Verification items for the finished model (mm, model axes). Face numbers are marked on the shaded views. A direction names the side the tool comes from. Coordinates: 2 decimals unless noted, no trailing zeros. Write each loop counter-clockwise with the first axis right and the second up, starting at its lowest first coordinate (ties: lowest second). Pieces come first, ordered by that corner, then holes. Notation, with made-up numbers: (-15.5, 77.5) -> (28.5, 77.5) arc R24 ccw to (28.5, 89.5) -> close; hole circle Ø3 at (8.5, -25). An arc over 180 degrees is marked (long way). Answer in a Markdown table with one row per item.
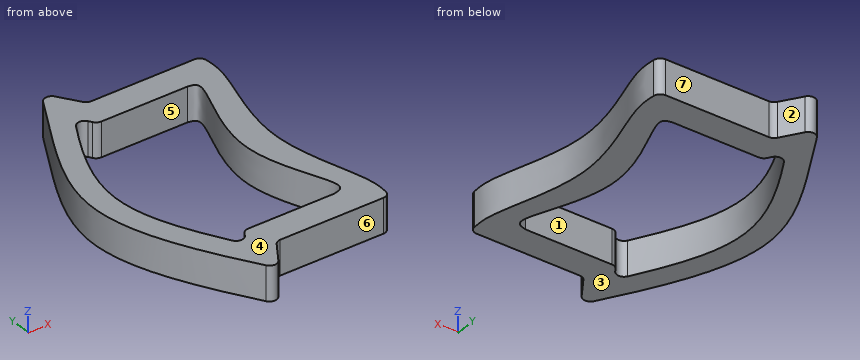
```python
from build123d import *

# Parameters (mm, degrees)
F1_DEPTH = 19.05
F3_DEPTH = 19.05
F4_R     = 4


with BuildPart() as f1:
    # F0 (on Top) → F1 (new body)
    with BuildSketch(Plane.XY):
        with BuildLine():
            add(Edge.make_bspline(
                [(0, -88.9), (-18.7615667395, -58.872751179), (-55.497587887, 2.319356984), (-18.3044684192, 54.234037211), (0, 88.9)],
                knots=[0, 0, 0, 0, 0.5, 1, 1, 1, 1], degree=3))
            Line((0, -88.9), (12.096735135, -70.5242279326))
            Line((12.096735135, -70.5242279326), (75.096735135, -70.5242279326))
            add(Edge.make_bspline(
                [(75.096735135, 70.5242279326), (75.6453777141, 65.842621729), (77.7669512859, 52.4624280909), (54.0778767649, 0.0958361046), (77.7020868907, -53.1321501243), (75.6250650534, -66.0721629988), (75.096735135, -70.5242279326)],
                knots=[0, 0, 0, 0, 0.1764310118, 0.500837432, 0.8270944973, 1, 1, 1, 1], degree=3))
            Line((75.096735135, 70.5242279326), (12.096735135, 70.5242279326))
            Line((12.096735135, 70.5242279326), (0, 88.9))
        make_face()
    extrude(amount=F1_DEPTH)

    # F2 (on face) → F3 (cut)
    with BuildSketch(Plane.XY.offset(19.05)):
        with BuildLine():
            add(Edge.make_bspline(
                [(0, -63.9), (-15.0066513258, -38.561437128), (-33.4891316908, -0.0640391576), (-15.0195212491, 38.6895154432), (0, 63.9)],
                knots=[0, 0, 0, 0, 0.5, 1, 1, 1, 1], degree=3))
            Line((0, -63.9), (6.0483675675, -54.7121139663))
            Line((6.0483675675, -54.7121139663), (56.0483675675, -54.7121139663))
            add(Edge.make_bspline(
                [(55.7842407716, 54.5435819516), (57.8413429651, 54.264139175), (66.4918207205, 53.0890329839), (32.3838227626, -0.5635362626), (68.3251031662, -51.8911242436), (58.5903282755, -54.1280136592), (56.0483675675, -54.7121139663)],
                knots=[0, 0, 0, 0, 0.1173857138, 0.4936276425, 0.8677752027, 1, 1, 1, 1], degree=3))
            Line((55.7842407716, 54.5435819516), (5.7842407716, 54.5435819516))
            Line((5.7842407716, 54.5435819516), (0, 63.9))
        make_face()
    extrude(amount=-F3_DEPTH, mode=Mode.SUBTRACT)

    # F4
    f4_edges = [f1.edges().sort_by_distance(p)[0] for p in [
        (0, -88.9, 9.525),
        (75.096735, -70.524228, 9.525),
        (5.784241, 54.543582, 9.525),
        (75.096735, 70.524228, 9.525),
        (0, 88.9, 9.525),
        (12.096735, 70.524228, 9.525),
        (12.096735, -70.524228, 9.525),
        (0, 63.9, 9.525),
        (0, -63.9, 9.525),
        (6.048368, -54.712114, 9.525),
    ]]
    fillet(f4_edges, radius=F4_R)


solid = f1.part
```
1. Go/stop test with flat-tipped pins: pin 1 (1.5 mm diameter, centred on y = 28.5, z = 14, fed in from +X); pin 2 (6 mm diameter, centred on y = -17.5, z = 9.5, fed in from -X); pin 3 (8 mm diameter, centred on y = -4.5, z = 2, fed in from +X). Record where each tip stops, or that it passes through.
Findings below:
| item | result |
|---|---|
| pin 1 | stops at x = 68.14 |
| pin 2 | stops at x = -35.58 |
| pin 3 | stops at x = 63.87 |
2. Material ranges on probe 1 along X at (y, z) = (1, 18); probe 2 along Y at (x, z) = (24.5, 3.25); probe 3 along X at (y, z) = (32, 14), recorded low to high. Write a range as from..to.
Findings below:
| item | result |
|---|---|
| probe 1 | x = -37..-24.24, 47.39..63.41 |
| probe 2 | y = -70.52..-54.71, 54.54..70.52 |
| probe 3 | x = -29.84..-16.83, 54.28..68.92 |
3. Access from +Z, -Z, +X, -X, +Y, -Y to the whole of each face (thin tool, end or side, straight path). Record for the marked faces 4, 5, 6 and 7.
Findings below:
| item | result |
|---|---|
| face 4 | +Z, +X, -X, +Y, -Y |
| face 5 | +Z, -Z |
| face 6 | +Z, -Z, +X, -Y |
| face 7 | +Z, -Z, +X, +Y |
4. Release check for a two-part mould opening along Y. For the marked faces 1, 2 and 3 record: released by +Y, released by -Y, zero draft, split by the parting line, or undercut.
Findings below:
| item | result |
|---|---|
| face 1 | undercut |
| face 2 | released by +Y |
| face 3 | zero draft |
5. Sectioned sample at A-A, the plane x = 21. Record the cut outline in (y, z).
Findings below:
| item | result |
|---|---|
| outline | (-70.52, 0) -> (-54.71, 0) -> (-54.71, 19.05) -> (-70.52, 19.05) -> close; (54.54, 0) -> (70.52, 0) -> (70.52, 19.05) -> (54.54, 19.05) -> close |
